Here's how the part is built. I have some questions about the finished solid (model axes, mm). Face numbers are marked on the shaded views. A direction names the side the tool comes from. Coordinates: 2 decimals unless noted, no trailing zeros. Order: outer loops, then holes, each group sorted by start corner. A loop starts at its lowest first (then second) coordinate and runs counter-clockwise, first axis right, second up. Notation, with made-up numbers: (0.25, 10.5) - (49.25, 10.5) arc R18 ccw to (49.25, 37.5) - close; hole circle Ø2 at (32, -30). An arc over 180 degrees is marked (long way). Answer as CSV lines item,"result". Start each with the question number.
Item 1: On a 3-axis mill with a long thin cutter (end or side, diameter ignored), from which of +Z, -Z, +X, -X, +Y, -Y can I reach the whole of each face in a straight line? I mean the marked faces 4 and 5. Say none if no direction works.
Item 2: Imagine slicing it at B-B on x = 14.5. List the corners of the cut face in (y, z) for me (3 decimals).
Item 3: We'd pull the mould along Y, two halves only. Please class the marked faces 1, 2 and 3: pulls with the +Y half, pulls with the -Y half, needs draft (parallel to the pull), parting line crosses it, or undercut.
Item 4: Imagine slicing it at A-A on y = 56. List the corners of the cut face in (x, z) for me, and give its area (3 significant figures).
Item 5: I'm going to push flat-ended pins straight in: pin 1 (9.5 mm diameter, centred on x = -17, z = 15.5, fed in from -Y); pin 2 (7.5 mm diameter, centred on y = -3, z = 17.5, fed in from +X); pin 3 (8 mm diameter, centred on y = 57, z = 13, fed in from -X). Where does each tip first touch, or does it pass through?
Item 6: Imagine slicing it at D-D on x = -19.5. List the corners of the cut face in (y, z) for me (3 decimals), and give its area (3 significant figures).
Item 7: Imagine slicing it at C-C on z = 9.75. Count the separate pieces of the cut face and the enclosed holes in it, and give its area (3 significant figures).
Item 8: I need wall thicknesses on line 1 (Y direction, x = 9.5, z = 14.5) (3 decimals); line 2 (X direction, y = 33.5, z = 18); line 3 (Y direction, x = -18.5, z = 18) (3 decimals). Which ranges of each line are inside material? Lowest first, please.
from build123d import *

# Parameters (mm, degrees)
F0_W     = 27.94
F0_H     = 139.7
F0_W_2   = 19.05
F0_H_2   = 19.05
F0_H_3   = 16.3293534029
F0_W_3   = 7.62
F1_DEPTH = 25.4
F2_W     = 64.4415542483
F2_H     = 139.5248323679
F3_DEPTH = 6.35


with BuildPart() as f1:
    # F0 (on Top) → F1 (new body)
    with BuildSketch(Plane.XY):
        with Locations((-17.78, 0)):
            Rectangle(F0_W, F0_H)
        with Locations((-18.415, -52.705)):
            Rectangle(F0_W_2, F0_H_2, mode=Mode.SUBTRACT)
        with Locations((-18.415, -28.575)):
            Rectangle(F0_W_2, F0_H_2, mode=Mode.SUBTRACT)
        with Locations((-18.415, 6.35)):
            Rectangle(F0_W_2, F0_H_2, mode=Mode.SUBTRACT)
        with Locations((-18.415, 30.5456899792)):
            Rectangle(F0_W_2, F0_H_2, mode=Mode.SUBTRACT)
        with Locations((-18.415, 54.0653232986)):
            Rectangle(F0_W_2, F0_H_3, mode=Mode.SUBTRACT)
        Rectangle(F0_W_3, F0_H)
        with Locations((17.78, 0)):
            Rectangle(F0_W, F0_H)
        with Locations((17.145, -54.2791421771)):
            Rectangle(F0_W_2, F0_H_2, mode=Mode.SUBTRACT)
        with Locations((17.145, -24.7503119767)):
            Rectangle(F0_W_2, F0_H_2, mode=Mode.SUBTRACT)
        with Locations((17.145, 6.35)):
            Rectangle(F0_W_2, F0_H_2, mode=Mode.SUBTRACT)
        with Locations((17.145, 29.1921038866)):
            Rectangle(F0_W_2, F0_H_2, mode=Mode.SUBTRACT)
        with Locations((17.145, 52.705)):
            Rectangle(F0_W_2, F0_H_2, mode=Mode.SUBTRACT)
    extrude(amount=F1_DEPTH)

    # F2 (on Top) → F3 (join)
    with BuildSketch(Plane.XY):
        with Locations((0.0985339284, -0.1970678568)):
            Rectangle(F2_W, F2_H)
    extrude(amount=F3_DEPTH)


solid = f1.part
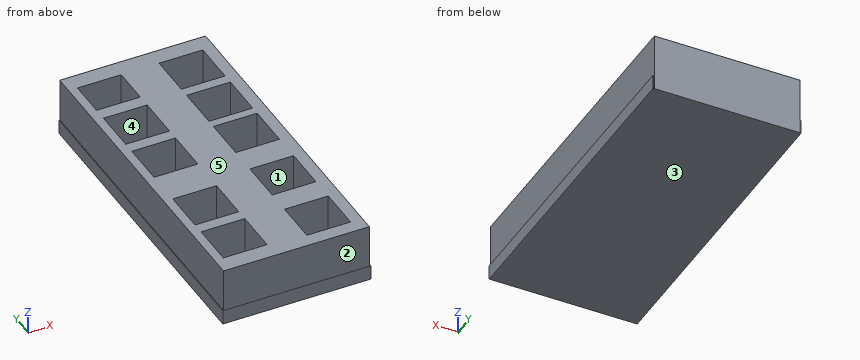
Responses:
1,face 4,"+Z"
1,face 5,"+Z, +X, -X, +Y, -Y"
2,outline,"(-69.959, 0) - (69.85, 0) - (69.85, 25.4) - (62.23, 25.4) - (62.23, 6.35) - (43.18, 6.35) - (43.18, 25.4) - (38.717, 25.4) - (38.717, 6.35) - (19.667, 6.35) - (19.667, 25.4) - (15.875, 25.4) - (15.875, 6.35) - (-3.175, 6.35) - (-3.175, 25.4) - (-15.225, 25.4) - (-15.225, 6.35) - (-34.275, 6.35) - (-34.275, 25.4) - (-44.754, 25.4) - (-44.754, 6.35) - (-63.804, 6.35) - (-63.804, 25.4) - (-69.85, 25.4) - (-69.85, 6.35) - (-69.959, 6.35) - close"
3,face 1,"undercut"
3,face 2,"pulls with the -Y half"
3,face 3,"needs draft"
4,outline,"(-32.12, 0) - (32.32, 0) - (32.32, 6.35) - (31.75, 6.35) - (31.75, 25.4) - (26.67, 25.4) - (26.67, 6.35) - (7.62, 6.35) - (7.62, 25.4) - (-8.89, 25.4) - (-8.89, 6.35) - (-27.94, 6.35) - (-27.94, 25.4) - (-31.75, 25.4) - (-31.75, 6.35) - (-32.12, 6.35) - close"
4,area,"893 mm^2"
5,pin 1,"stops at y = -69.85"
5,pin 2,"stops at x = 31.75"
5,pin 3,"stops at x = -31.75"
6,outline,"(-69.959, 0) - (69.85, 0) - (69.85, 25.4) - (62.23, 25.4) - (62.23, 6.35) - (45.901, 6.35) - (45.901, 25.4) - (40.071, 25.4) - (40.071, 6.35) - (21.021, 6.35) - (21.021, 25.4) - (15.875, 25.4) - (15.875, 6.35) - (-3.175, 6.35) - (-3.175, 25.4) - (-19.05, 25.4) - (-19.05, 6.35) - (-38.1, 6.35) - (-38.1, 25.4) - (-43.18, 25.4) - (-43.18, 6.35) - (-62.23, 6.35) - (-62.23, 25.4) - (-69.85, 25.4) - (-69.85, 6.35) - (-69.959, 6.35) - close"
6,area,"1,790 mm^2"
7,separate pieces,"1"
7,enclosed holes,"10"
7,area,"5,290 mm^2"
8,line 1,"y = -69.85 to -63.804, -44.754 to -34.275, -15.225 to -3.175, 15.875 to 19.667, 38.717 to 43.18, 62.23 to 69.85"
8,line 2,"x = -31.75 to -27.94, -8.89 to 7.62, 26.67 to 31.75"
8,line 3,"y = -69.85 to -62.23, -43.18 to -38.1, -19.05 to -3.175, 15.875 to 21.021, 40.071 to 45.901, 62.23 to 69.85"
